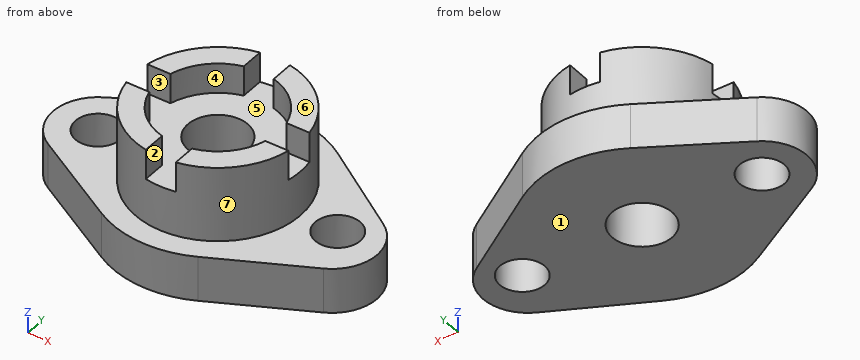
```python
from build123d import *

# Parameters (mm, degrees)
F0_R     = 9.525
F0_R_2   = 34.925
F1_DEPTH = 19.05
F0_R_3   = 25.4
F2_DEPTH = 50.8
F0_R_4   = 12.7
F3_DEPTH = 38.1
F5_DEPTH = 12.7
F7_DEPTH = 12.7


with BuildPart() as f1:
    # F0 (on Top) → F1 (new body)
    with BuildSketch(Plane.XY):
        with BuildLine():
            Line((-60.325, -16.4977839421), (-22.225, -38.4948291982))
            ThreePointArc((-22.225, -38.4948291982), (-1.4272180614, -44.4270812524), (19.7084347148, -39.8419389725))
            Line((19.7084347148, -39.8419389725), (59.1417276134, -20.3356473933))
            ThreePointArc((59.1417276134, -20.3356473933), (69.70597644, -4.4832296998), (61.2595044194, 12.5918870027))
            Line((61.2595044194, 12.5918870027), (24.6499139288, 36.9889746181))
            ThreePointArc((24.6499139288, 36.9889746181), (1.4272180614, 44.4270812524), (-22.225, 38.4948291982))
            Line((-22.225, 38.4948291982), (-60.325, 16.4977839421))
            ThreePointArc((-60.325, 16.4977839421), (-69.85, 0), (-60.325, -16.4977839421))
        make_face()
        with Locations((-50.8, 0)):
            Circle(F0_R, mode=Mode.SUBTRACT)
        Circle(F0_R_2, mode=Mode.SUBTRACT)
        with Locations((50.8, 0)):
            Circle(F0_R, mode=Mode.SUBTRACT)
    extrude(amount=F1_DEPTH)

    # F0 (on Top) → F2 (join)
    with BuildSketch(Plane.XY):
        Circle(F0_R_2)
        Circle(F0_R_3, mode=Mode.SUBTRACT)
    extrude(amount=F2_DEPTH)

    # F0 (on Top) → F3 (join)
    with BuildSketch(Plane.XY):
        Circle(F0_R_3)
        Circle(F0_R_4, mode=Mode.SUBTRACT)
    extrude(amount=F3_DEPTH)

    # F4 (on face) → F5 (cut)
    with BuildSketch(Plane.XY.offset(50.8)):
        with BuildLine():
            ThreePointArc((6.35, 34.3428758988), (0, 34.925), (-6.35, 34.3428758988))
            Line((-6.35, 34.3428758988), (-6.35, 24.5934442484))
            ThreePointArc((-6.35, 24.5934442484), (0, 25.4), (6.35, 24.5934442484))
            Line((6.35, 24.5934442484), (6.35, 34.3428758988))
        make_face()
    extrude(amount=-F5_DEPTH, mode=Mode.SUBTRACT)

    # F6 (on face) → F7 (cut)
    with BuildSketch(Plane.XY.offset(50.8)):
        with BuildLine():
            Line((-24.5934442484, 6.35), (-34.3428758988, 6.35))
            ThreePointArc((-34.3428758988, 6.35), (-34.925, 0), (-34.3428758988, -6.35))
            Line((-34.3428758988, -6.35), (-24.5934442484, -6.35))
            ThreePointArc((-24.5934442484, -6.35), (-25.4, 0), (-24.5934442484, 6.35))
        make_face()
        with BuildLine():
            Line((-6.35, -24.5934442484), (-6.35, -34.3428758988))
            ThreePointArc((-6.35, -34.3428758988), (0, -34.925), (6.35, -34.3428758988))
            Line((6.35, -34.3428758988), (6.35, -24.5934442484))
            ThreePointArc((6.35, -24.5934442484), (0, -25.4), (-6.35, -24.5934442484))
        make_face()
        with BuildLine():
            Line((24.5934442484, -6.35), (34.3428758988, -6.35))
            ThreePointArc((34.3428758988, -6.35), (34.7791644937, -3.1883133656), (34.925, 0))
            ThreePointArc((34.925, 0), (34.7791644937, 3.1883133656), (34.3428758988, 6.35))
            Line((34.3428758988, 6.35), (24.5934442484, 6.35))
            ThreePointArc((24.5934442484, 6.35), (25.4, 0), (24.5934442484, -6.35))
        make_face()
    extrude(amount=-F7_DEPTH, mode=Mode.SUBTRACT)


solid = f1.part
```
For this review, take the finished solid that the model builds, in its own axes (mm). Face numbers are marked on the shaded views. A direction names the side the tool comes from. Round coordinates to 2 decimals unless told otherwise and drop trailing zeros. Write each loop counter-clockwise with the first axis right and the second up, starting at its lowest first coordinate (ties: lowest second). Pieces come first, ordered by that corner, then holes. Notation, with made-up numbers: (55, 89) -> (107, 89) arc R13 cw to (107, 109) -> close; hole circle Ø3 at (70.25, 25.5). An arc over 180 degrees is marked (long way). One line per question, with ' | ' between items. Start each with the question number.
1) For pin 1 Ø5 at (x, z) = (-39.5, 23.5) entering from +Y; pin 2 Ø8 at (x, z) = (-31.5, 47.5) entering from +Y; pin 3 Ø5 at (y, z) = (-30, 47.5) entering from +X; pin 4 Ø4 at (x, z) = (-3.5, 31) entering from +Y, all flat-tipped, find the tip position at first contact; note any pin that passes through.
2) Wall thickness on line 1 along Y through (x, z) = (0, 21.5) (3 decimals); line 2 along Z through (x, y) = (-61, 8); line 3 along Z through (x, y) = (-6, 17.5): over which ranges is each line inside the solid? List them lowest first.
3) Add section C-C (z = 45). Write out the cut boundary in (x, y) (3 decimals), and give its area (3 significant figures).
4) Machinability: for the marked faces 1, 2 and 3, which of the approach directions +Z, -Z, +X, -X, +Y, -Y give a long, thin tool a straight path to every point of the face, cutting with its end or side? Answer none if there is none.
5) Mouldability with a two-part tool opening along Y and no side actions: class the marked faces 4, 5, 6 and 7 as +Y half, -Y half, draft (parallel to the pull), parting line (faces both ways), or undercut.
6) Add section B-B (z = 5.5). Count the separate pieces of the cut face and the enclosed holes in it, and give its area (3 significant figures).
7) Add section A-A (x = 0). Write out the cut boundary in (y, z) (3 decimals), and give its area (3 significant figures).
8) Add section D-D (y = 0). Write out the cut boundary in (x, z) (3 decimals).
Reported:
1) pin 1: passes through | pin 2: stops at y = 21.53 | pin 3: stops at x = 21.53 | pin 4: stops at y = 34.89
2) line 1: y = -34.925 to -12.7, 12.7 to 34.925 | line 2: z = 0 to 19.05 | line 3: z = 0 to 38.1
3) outline: (-34.343, -6.35) arc R34.925 ccw to (-6.35, -34.343) -> (-6.35, -24.593) arc R25.4 cw to (-24.593, -6.35) -> close; (-34.343, 6.35) -> (-24.593, 6.35) arc R25.4 cw to (-6.35, 24.593) -> (-6.35, 34.343) arc R34.925 ccw to start; (6.35, -34.343) arc R34.925 ccw to (34.343, -6.35) -> (24.593, -6.35) arc R25.4 cw to (6.35, -24.593) -> close; (6.35, 24.593) arc R25.4 cw to (24.593, 6.35) -> (34.343, 6.35) arc R34.925 ccw to (6.35, 34.343) -> close | area: 1,320 mm²
4) face 1: -Z, +X, -X, +Y, -Y | face 2: +Z, +Y, -Y | face 3: +Z, +X, -X
5) face 4: undercut | face 5: undercut | face 6: draft | face 7: parting line
6) separate pieces: 1 | enclosed holes: 3 | area: 7,340 mm²
7) outline: (-44.45, 0) -> (-12.7, 0) -> (-12.7, 38.1) -> (-34.925, 38.1) -> (-34.925, 19.05) -> (-44.45, 19.05) -> close; (12.7, 0) -> (44.45, 0) -> (44.45, 19.05) -> (34.925, 19.05) -> (34.925, 38.1) -> (12.7, 38.1) -> close | area: 2,060 mm²
8) outline: (-69.85, 0) -> (-60.325, 0) -> (-60.325, 19.05) -> (-69.85, 19.05) -> close; (-41.275, 0) -> (-12.7, 0) -> (-12.7, 38.1) -> (-34.925, 38.1) -> (-34.925, 19.05) -> (-41.275, 19.05) -> close; (12.7, 0) -> (41.275, 0) -> (41.275, 19.05) -> (34.925, 19.05) -> (34.925, 38.1) -> (12.7, 38.1) -> close; (60.325, 0) -> (69.464, 0) -> (69.464, 19.05) -> (60.325, 19.05) -> close
